CAD build for the part. Positions are in the model's coordinates, mm. Face numbers are marked on the shaded views. A direction names the side the tool comes from. Round coordinates to 2 decimals unless told otherwise and drop trailing zeros. Loops run counter-clockwise (first coordinate to the right, second up) from the corner with the lowest first, then second, coordinate; pieces in that order, holes last.
```python
from build123d import *

# Parameters (mm, degrees)
ESQUISSE1_W             = 272.524799983
ESQUISSE1_H             = 173.408070163
ESQUISSE1_R             = 6
BOSS_EXTRU_1_DEPTH      = 5
ESQUISSE2_OUTSIDE_W     = 339.137
ESQUISSE2_OUTSIDE_H     = 240.02
ENL_V_MAT_EXTRU_1_DEPTH = 5
BOSS_EXTRU_2_DEPTH      = 80
ESQUISSE4_R             = 6
ENL_V_MAT_EXTRU_2_DEPTH = 98.574759668
BOSS_EXTRU_3_DEPTH      = 2.5


with BuildPart() as part:
    # Esquisse1 → Boss.-Extru.1 (new body)
    with BuildSketch(Plane.XY):
        with Locations((-544.151755804, 61.14332382)):
            Rectangle(ESQUISSE1_W, ESQUISSE1_H)
        with Locations((-580.420844254, 0.36763792)):
            Circle(ESQUISSE1_R, mode=Mode.SUBTRACT)
        with Locations((-480.421520044, 0)):
            Circle(ESQUISSE1_R, mode=Mode.SUBTRACT)
        with Locations((-530, 114.747437119)):
            Circle(ESQUISSE1_R, mode=Mode.SUBTRACT)
    extrude(amount=BOSS_EXTRU_1_DEPTH)

    # Esquisse2 outside → Enlèv. mat.-Extru.1 (cut)
    with BuildSketch(Plane.XY.offset(5)):
        with Locations((-544.1515, 61.143)):
            Rectangle(ESQUISSE2_OUTSIDE_W, ESQUISSE2_OUTSIDE_H)
        with BuildLine():
            Line((-534.956009313, 134.12365893), (-627.481332722, 110.457726071))
            ThreePointArc((-627.481332722, 110.457726071), (-643.319491193, 97.095160735), (-642.680296555, 76.382921688))
            Line((-642.680296555, 76.382921688), (-598.149058477, -8.890354328))
            ThreePointArc((-598.149058477, -8.890354328), (-590.816634727, -16.718249252), (-580.494371838, -19.632226922))
            Line((-580.494371838, -19.632226922), (-480.495047628, -19.999864842))
            ThreePointArc((-480.495047628, -19.999864842), (-463.728705311, -11.015894711), (-462.061930105, 7.932556793))
            Line((-462.061930105, 7.932556793), (-511.640410061, 122.679993912))
            ThreePointArc((-511.640410061, 122.679993912), (-521.187885573, 132.701451693), (-534.956009313, 134.12365893))
        make_face(mode=Mode.SUBTRACT)
    extrude(amount=-ENL_V_MAT_EXTRU_1_DEPTH, mode=Mode.SUBTRACT)

    # Esquisse3 → Boss.-Extru.2 (add)
    with BuildSketch(Plane.XY.offset(5)):
        Polygon((-586.213116183, 77.574759668), (-506.213116183, 77.574759668), (-506.213116183, 72.574759668), (-581.213116183, 72.574759668), (-581.213116183, 22.574759668), (-506.213116183, 22.574759668), (-506.213116183, 17.574759668), (-586.213116183, 17.574759668), (-586.213116183, 22.574759668), (-586.213116183, 72.574759668), align=None)
    extrude(amount=BOSS_EXTRU_2_DEPTH)

    # Esquisse4 → Enlèv. mat.-Extru.2 (cut, through all)
    with BuildSketch(Plane(origin=(0, 77.574759668, 0), x_dir=(1, 0, 0), z_dir=(0, 1, 0))):
        with Locations(Location((-546.213116183, -70, 0), (0, 0, 270))):  # turned: the seam where the file's is
            Circle(ESQUISSE4_R)
    extrude(amount=-ENL_V_MAT_EXTRU_2_DEPTH, mode=Mode.SUBTRACT)

    # Esquisse5 → Boss.-Extru.3 (add, symmetric)
    with BuildSketch(Plane.ZY.offset(546.213116183)):
        Polygon((5, 107.574759668), (40, 77.574759668), (5, 77.574759668), align=None)
        Polygon((5, 17.574759668), (5, -12.425240332), (40, 17.574759668), align=None)
    extrude(amount=BOSS_EXTRU_3_DEPTH, both=True)


solid = part.part
```
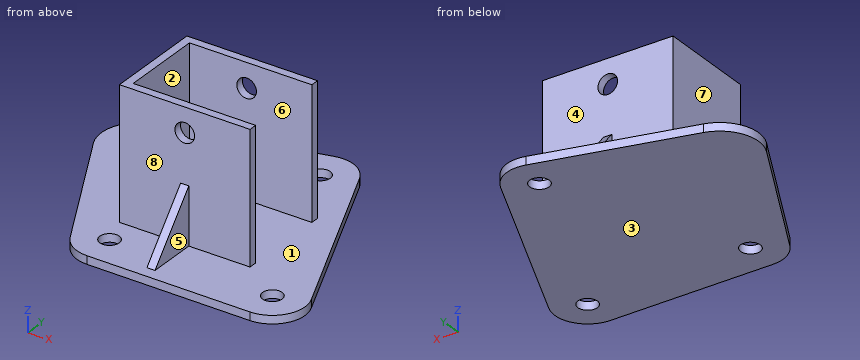
Item 1: Cut at C-C, the plane y = 45. Give the cut face in (x, z), plus the area to 3 significant figures.
Answers follow:
outline: (-626.29, 0) - (-478.08, 0) - (-478.08, 5) - (-581.21, 5) - (-581.21, 85) - (-586.21, 85) - (-586.21, 5) - (-626.29, 5) - close
area: 1,140 mm2
Item 2: Probe line 1 (X direction, y = 19.95, z = 70); line 2 (Y direction, x = -520, z = 27); line 3 (Y direction, x = -544, z = 32). List the from-to ranges inside material, lowest first.
Answers follow:
line 1: x = -586.21 to -552.21, -540.21 to -506.21
line 2: y = 17.57 to 22.57, 72.57 to 77.57
line 3: y = 10.72 to 22.57, 72.57 to 84.43
Item 3: Flat gauge pins, fed straight in: P1, Ø1, axis at x = -585, z = 63.5, coming from the -Y side; P2, Ø4, axis at x = -555, z = 51, coming from the +Y side; P3, Ø11, axis at x = -580.42, y = 0.37, coming from the -Z side; P4, Ø15, axis at y = 6.5, z = 14.5, coming from the -X side. Where does each tip first touch, or does it go through?
Answers follow:
P1: stops at y = 17.57
P2: stops at y = 77.57
P3: passes through
P4: stops at x = -548.71
Item 4: Cut at A-A, the plane z = 70. Give the cut face in (x, y), plus the area to 3 significant figures.
Answers follow:
outline: (-586.21, 17.57) - (-552.21, 17.57) - (-552.21, 22.57) - (-581.21, 22.57) - (-581.21, 72.57) - (-552.21, 72.57) - (-552.21, 77.57) - (-586.21, 77.57) - close; (-540.21, 17.57) - (-506.21, 17.57) - (-506.21, 22.57) - (-540.21, 22.57) - close; (-540.21, 72.57) - (-506.21, 72.57) - (-506.21, 77.57) - (-540.21, 77.57) - close
area: 930 mm2
Item 5: Cut at B-B, the plane x = -484. Give the cut face in (y, z), plus the area to 3 significant figures.
Answers follow:
outline: (-19.99, 0) - (-4.82, 0) - (-4.82, 5) - (-19.99, 5) - close; (4.82, 0) - (58.71, 0) - (58.71, 5) - (4.82, 5) - close
area: 345 mm2
Item 6: Two-plate mould, pull along Y, no slides. Class the marked faces 1, 2, 3 and 4: released by +Y, released by -Y, zero draft, split by the parting line, or undercut.
Answers follow:
face 1: undercut
face 2: undercut
face 3: zero draft
face 4: released by +Y
Item 7: 3-axis set-ups, long thin cutter, end or side, ignore diameter. For the marked faces 5, 6, 7 and 8: which of +Z, -Z, +X, -X, +Y, -Y reach the whole face in a straight line?
Answers follow:
face 5: +Z, +X, -Y
face 6: +Z, +X
face 7: +Z, -X, +Y, -Y
face 8: +Z, -Y
Item 8: Cut at D-D, the plane x = -530. Give the cut face in (y, z), plus the area to 3 significant figures.
Answers follow:
outline: (-19.82, 0) - (108.75, 0) - (108.75, 5) - (77.57, 5) - (77.57, 85) - (72.57, 85) - (72.57, 5) - (22.57, 5) - (22.57, 85) - (17.57, 85) - (17.57, 5) - (-19.82, 5) - close; (120.75, 0) - (134.75, 0) - (134.75, 5) - (120.75, 5) - close
area: 1,510 mm2
